CAD build for the part. Positions are in the model's coordinates, mm. Face numbers are marked on the shaded views. Coordinates: 2 decimals unless noted, no trailing zeros. Write each loop counter-clockwise with the first axis right and the second up, starting at its lowest first coordinate (ties: lowest second). Pieces come first, ordered by that corner, then holes. Notation, with made-up numbers: (5, -17.5) -> (43, -17.5) arc R16 ccw to (43, 13.5) -> close; hole circle Ø3 at (33, -23). An arc over 180 degrees is marked (long way). Answer as CSV lines item,"result".
```python
from build123d import *

# Parameters (mm, degrees)
VERRUNDUNG1_R = 20
VERRUNDUNG4_R = 10
VERRUNDUNG5_R = 10


with BuildPart() as part:
    # Skizze1 → Rotation1 (revolve)
    with BuildSketch(Plane.XY):
        Polygon((0, 0), (25, 0), (25, 178), (14, 178), (14, 200), (10, 200), (10, 177), (13, 177), (24, 177), (24, 1), (0, 1), align=None)
    revolve(axis=Axis((0, 0, 0), (0, 1, 0)))

    # Verrundung1
    verrundung1_edges = [part.edges().sort_by_distance(p)[0] for p in [
        (-25, 0, 0),
        (-24, 1, 0),
    ]]
    fillet(verrundung1_edges, radius=VERRUNDUNG1_R)

    # Verrundung4
    verrundung4_edges = [part.edges().sort_by_distance(p)[0] for p in [
        (-25, 178, 0),
        (-24, 177, 0),
    ]]
    fillet(verrundung4_edges, radius=VERRUNDUNG4_R)

    # Verrundung5
    verrundung5_edges = [part.edges().sort_by_distance(p)[0] for p in [
        (-14, 178, 0),
        (-10, 177, 0),
    ]]
    fillet(verrundung5_edges, radius=VERRUNDUNG5_R)


solid = part.part
```
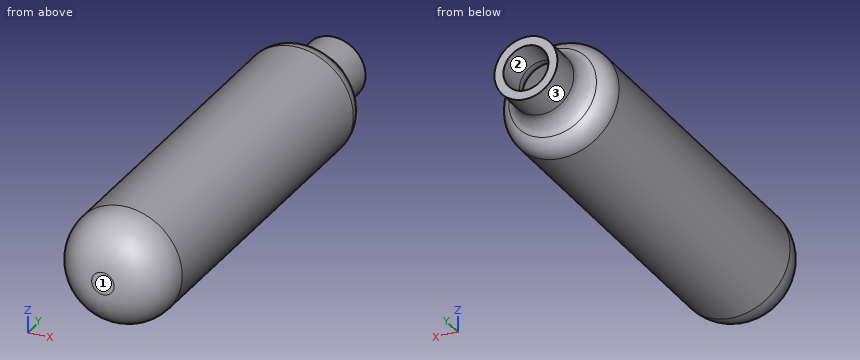
Item 1: Saw through at B-B on y = 172. Give the cut face in (x, z), and give its area (3 significant figures).
Answer below:
outline,"circle Ø48.33 at (0, 0); hole circle Ø45.32 at (0, 0)"
area,"221 mm2"
Item 2: Saw through at A-A on y = 111. Give the cut face in (x, z).
Answer below:
outline,"circle Ø50 at (0, 0); hole circle Ø48 at (0, 0)"
Item 3: Flat gauge pins, fed straight in: pin 1 (5 mm diameter, centred on y = 75, z = 17, fed in from +X); pin 2 (1.5 mm diameter, centred on x = -6.5, z = 10, fed in from -Y); pin 3 (2 mm diameter, centred on y = 79, z = -18, fed in from -X). Where does each tip first touch, or does it go through?
Answer below:
pin 1,"stops at x = 20.37"
pin 2,"stops at y = 0.98"
pin 3,"stops at x = -18.33"
Item 4: Two-plate mould, pull along Z, no slides. Class the marked faces 1, 2 and 3: pulls with the +Z half, pulls with the -Z half, needs draft (parallel to the pull), parting line crosses it, or undercut.
Answer below:
face 1,"needs draft"
face 2,"undercut"
face 3,"parting line crosses it"
Item 5: Wall check: line 1 (Z direction, x = 0, y = 64.5); line 2 (Z direction, x = 0, y = 194). Give the ranges that are in metal, low to high. Write a range as from..to.
Answer below:
line 1,"z = -25..-24, 24..25"
line 2,"z = -14..-10, 10..14"
